```python
from build123d import *

# Parameters (mm, degrees)
SKETCH1_W               = 120
SKETCH1_H               = 108
BOSS_EXTRUDE1_DEPTH     = 11
SKETCH4_W               = 114
SKETCH4_H               = 102
CUT_EXTRUDE1_DEPTH      = 8
SKETCH6_R               = 1.999999993
SKETCH6_R_2             = 2
CUT_EXTRUDE6_DEPTH      = 118
CUT_EXTRUDE6_DEPTH_BACK = 4
SKETCH5_R               = 2
CUT_EXTRUDE5_DEPTH      = 106
CUT_EXTRUDE5_DEPTH_BACK = 4
FILLET2_R               = 1


with BuildPart() as part:
    # Sketch1 → Boss-Extrude1 (new body)
    with BuildSketch(Plane(origin=(0, 0, 0), x_dir=(1, 0, 0), z_dir=(0, 1, 0))):
        with Locations((-141.609907121, 23.894736842)):
            Rectangle(SKETCH1_W, SKETCH1_H)
    extrude(amount=BOSS_EXTRUDE1_DEPTH)

    # Sketch4 → Cut-Extrude1 (cut)
    with BuildSketch(Plane(origin=(0, 11, 0), x_dir=(1, 0, 0), z_dir=(0, 1, 0))):
        with Locations((-141.609907121, 23.894736842)):
            Rectangle(SKETCH4_W, SKETCH4_H)
    extrude(amount=-CUT_EXTRUDE1_DEPTH, mode=Mode.SUBTRACT)

    # Sketch6 → Cut-Extrude6 (cut, two sides)
    with BuildSketch(Plane(origin=(-198.609907121, 0, 0), x_dir=(0, 0, -1), z_dir=(1, 0, 0))) as cut_extrude6_sk:
        with Locations((-1.105263158, 6.999999977)):
            Circle(SKETCH6_R)
        with Locations((23.894736842, 6.999999977)):
            Circle(SKETCH6_R_2)
        with Locations((48.894736842, 7)):
            Circle(SKETCH6_R_2)
    extrude(amount=CUT_EXTRUDE6_DEPTH, mode=Mode.SUBTRACT)
    extrude(cut_extrude6_sk.sketch, amount=-CUT_EXTRUDE6_DEPTH_BACK, mode=Mode.SUBTRACT)

    # Sketch5 → Cut-Extrude5 (cut, two sides)
    with BuildSketch(Plane.XY.offset(-74.894736842)) as cut_extrude5_sk:
        with Locations((-170.859907121, 7)):
            Circle(SKETCH5_R)
        with Locations((-141.609907121, 7)):
            Circle(SKETCH5_R)
        with Locations((-112.359907121, 7)):
            Circle(SKETCH5_R)
    extrude(amount=CUT_EXTRUDE5_DEPTH, mode=Mode.SUBTRACT)
    extrude(cut_extrude5_sk.sketch, amount=-CUT_EXTRUDE5_DEPTH_BACK, mode=Mode.SUBTRACT)

    # Fillet2
    fillet2_edges = [part.edges().sort_by_distance(p)[0] for p in [
        (-81.609907121, 11, -23.894736842),
        (-141.609907121, 11, -77.894736842),
        (-198.609907121, 11, -23.894736842),
        (-141.609907121, 11, 27.105263158),
        (-84.609907121, 11, -23.894736842),
        (-141.609907121, 11, -74.894736842),
        (-201.609907121, 11, -23.894736842),
        (-141.609907121, 11, 30.105263158),
    ]]
    fillet(fillet2_edges, radius=FILLET2_R)


solid = part.part
```
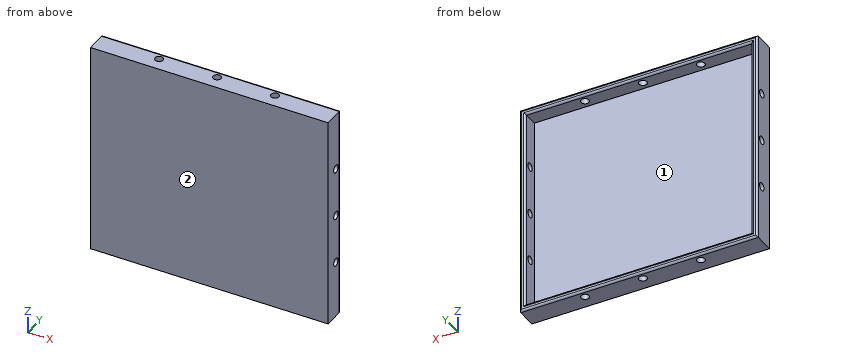
Source: CAD feature listing. Evaluate the final solid. Frame: model axes, mm. Face numbers are marked on the shaded views. Coordinates: 2 decimals unless noted, no trailing zeros. Write each loop counter-clockwise with the first axis right and the second up, starting at its lowest first coordinate (ties: lowest second). Pieces come first, ordered by that corner, then holes. Notation, with made-up numbers: (-16, 41.25) -> (40, 41.25) arc R15 ccw to (40, 55.25) -> close; hole circle Ø4 at (34, 33). An arc over 180 degrees is marked (long way). Return JSON: item names as keys, results as strings. Group by question number.
1) Mould query, pull axis X, two halves, no side actions, for the marked faces 1 and 2. Classes: +X half, -X half, draft (parallel to the pull), parting line (faces both ways), or undercut.
2) Section query D-D, the plane y = 7. State how many separate pieces and enclosed holes the cut face has, plus the area to 3 significant figures.
3) Section query C-C, the plane x = -126.5. Return loops of the section in (y, z).
4) Ray query, line 1 along Z through (x, y) = (-82.35, 7); line 2 along X through (y, z) = (9.75, -8.5); line 3 along X through (y, z) = (7, 28.1). Return the intervals inside material, ascending.
5) Section query B-B, the plane z = -18. Return loops of the section in (x, y), plus the area to 3 significant figures.
6) Contact query for a flat-ended pin moving along its axis: P1, Ø6, axis at x = -101, z = -58.5, coming from the +Y side. Output: stop coordinate, or through.
7) Section query A-A, the plane z = 1. Return loops of the section in (x, y).
From the geometry:
{
 "1": {"face 1": "undercut", "face 2": "draft"},
 "2": {"separate pieces": "12", "enclosed holes": "0", "area": "1,190 mm²"},
 "3": {"outline": "(0, -77.89) -> (10, -77.89) arc R1 ccw to (11, -76.89) -> (11, -75.89) arc R1 ccw to (10, -74.89) -> (3, -74.89) -> (3, 27.11) -> (10, 27.11) arc R1 ccw to (11, 28.11) -> (11, 29.11) arc R1 ccw to (10, 30.11) -> (0, 30.11) -> close"},
 "4": {"line 1": "-77.89 to -50.89, -46.89 to -25.89, -21.89 to -0.89, 3.11 to 30.11", "line 2": "-201.61 to -198.61, -84.61 to -81.61", "line 3": "-201.61 to -172.86, -168.86 to -143.61, -139.61 to -114.36, -110.36 to -81.61"},
 "5": {"outline": "(-201.61, 0) -> (-81.61, 0) -> (-81.61, 10) arc R1 ccw to (-82.61, 11) -> (-83.61, 11) arc R1 ccw to (-84.61, 10) -> (-84.61, 3) -> (-198.61, 3) -> (-198.61, 10) arc R1 ccw to (-199.61, 11) -> (-200.61, 11) arc R1 ccw to (-201.61, 10) -> close", "area": "407 mm²"},
 "6": {"P1": "y = 3"},
 "7": {"outline": "(-201.61, 0) -> (-81.61, 0) -> (-81.61, 5) -> (-84.61, 5) -> (-84.61, 3) -> (-198.61, 3) -> (-198.61, 5) -> (-201.61, 5) -> close; (-201.61, 9) -> (-198.61, 9) -> (-198.61, 10) arc R1 ccw to (-199.61, 11) -> (-200.61, 11) arc R1 ccw to (-201.61, 10) -> close; (-84.61, 9) -> (-81.61, 9) -> (-81.61, 10) arc R1 ccw to (-82.61, 11) -> (-83.61, 11) arc R1 ccw to (-84.61, 10) -> close"}
}
